Source: CAD feature listing. Evaluate the final solid. Frame: model axes, mm. A direction names the side the tool comes from. Round coordinates to 2 decimals unless told otherwise and drop trailing zeros. Loops run counter-clockwise (first coordinate to the right, second up) from the corner with the lowest first, then second, coordinate; pieces in that order, holes last.
Item 1: Section query B-B on y = 0. Return loops of the section in (x, z), then the cut area to 3 significant figures.
Item 2: Section query C-C on z = -16. Give the number of separate pieces and of enclosed holes in the cut face, then the cut area to 3 significant figures.
Item 3: Access query for faces 4 (the flat face through (10, 71, -21)), 5 (the flat face through (-3.965, 62.6, -27.4)), 6 (the flat face through (0, 3.965, -13)), 7 (the cylindrical face through (14.856, 165.986, -46.208)), 8 (the flat face through (-3.1, 70, -38)). Directions: +Z, -Z, +X, -X, +Y, -Y. A direction counts if a zero-diameter tool reaches every point of the face in a straight line with its end or side. Return the directions, or none.
Item 4: Pull-direction query (Z, two-part tool) for faces 1 (the flat face through (0, 164, -30)), 2 (the flat face through (7, 81, -20)), 3 (the flat face through (7, 10, -10)); classes: released by +Z, released by -Z, zero draft, split by the parting line, or undercut.
Item 5: Ray query, L1, parallel to Y at x = 0, z = -9.5; L2, parallel to Z at x = 9.5, y = 94; L3, parallel to Z at x = 0, y = 91. Return the intervals inside material, ascending.
Item 6: First-contact query: P1, Ø4.5, axis at x = -1, z = -19.5, coming from the +Y side; P2, Ø12, axis at y = 67.5, z = -28.5, coming from the +X side; P3, Ø2, axis at x = -1.5, z = -29.5, coming from the +Y side; P4, Ø21.5, axis at y = 58.5, z = -7, coming from the +X side. Flat tips, straight axial feed; report the tip coordinate or a pass-through.
Item 7: Section query A-A on x = 0. Return loops of the section in (y, z).
```python
from build123d import *

# Parameters (mm, degrees)
SKETCH2_R           = 2.5
SKETCH4_W           = 40
SKETCH4_H           = 40
BOSS_EXTRUDE1_DEPTH = 15
SKETCH5_R           = 10
CUT_EXTRUDE1_DEPTH  = 1
SKETCH6_R           = 2.5
BOSS_EXTRUDE2_DEPTH = 2


with BuildPart() as part:
    # Sweep1: sweep along a path in Sketch3
    with BuildLine(Plane(origin=(0, 0, 0), x_dir=(0, 0, -1), z_dir=(1, 0, 0))) as sweep1_path:
        Line((0, 0), (30, 0))
        Line((30, 0), (30, 150))
    # Sketch2 → Sweep1 (sweep)
    with BuildSketch(Plane.XY):
        with BuildLine():
            Line((-10, -10), (-3.1, -10))
            Line((-3.1, -10), (-3.1, -7.81857447))
            Line((-3.1, -7.81857447), (-4.285374034, -7.81857447))
            ThreePointArc((-4.285374034, -7.81857447), (-5.210402021, -7.198473435), (-4.988208383, -6.107220917))
            Line((-4.988208383, -6.107220917), (-2.819718275, -3.96470075))
            Line((-2.819718275, -3.96470075), (0, -3.96470075))
            Line((0, -3.96470075), (2.782738033, -3.96470075))
            Line((2.782738033, -3.96470075), (5.105242131, -6.103332486))
            ThreePointArc((5.105242131, -6.103332486), (5.359419929, -7.202533996), (4.427854938, -7.838959152))
            Line((4.427854938, -7.838959152), (3.1, -7.838959152))
            Line((3.1, -7.838959152), (3.1, -10))
            Line((3.1, -10), (10, -10))
            Line((10, -10), (10, -3.1))
            Line((10, -3.1), (7.81857447, -3.1))
            Line((7.81857447, -3.1), (7.81857447, -4.285374034))
            ThreePointArc((7.81857447, -4.285374034), (7.198473435, -5.210402021), (6.107220917, -4.988208383))
            Line((6.107220917, -4.988208383), (3.96470075, -2.819718275))
            Line((3.96470075, -2.819718275), (3.96470075, 0))
            Line((3.96470075, 0), (3.96470075, 2.782738033))
            Line((3.96470075, 2.782738033), (6.103332486, 5.105242131))
            ThreePointArc((6.103332486, 5.105242131), (7.202533996, 5.359419929), (7.838959152, 4.427854938))
            Line((7.838959152, 4.427854938), (7.838959152, 3.1))
            Line((7.838959152, 3.1), (10, 3.1))
            Line((10, 3.1), (10, 10))
            Line((10, 10), (3.1, 10))
            Line((3.1, 10), (3.1, 7.81857447))
            Line((3.1, 7.81857447), (4.285374034, 7.81857447))
            ThreePointArc((4.285374034, 7.81857447), (5.210402021, 7.198473435), (4.988208383, 6.107220917))
            Line((4.988208383, 6.107220917), (2.819718275, 3.96470075))
            Line((2.819718275, 3.96470075), (0, 3.96470075))
            Line((0, 3.96470075), (-2.782738033, 3.96470075))
            Line((-2.782738033, 3.96470075), (-5.105242131, 6.103332486))
            ThreePointArc((-5.105242131, 6.103332486), (-5.359419929, 7.202533996), (-4.427854938, 7.838959152))
            Line((-4.427854938, 7.838959152), (-3.1, 7.838959152))
            Line((-3.1, 7.838959152), (-3.1, 10))
            Line((-3.1, 10), (-10, 10))
            Line((-10, 10), (-10, 3.1))
            Line((-10, 3.1), (-7.81857447, 3.1))
            Line((-7.81857447, 3.1), (-7.81857447, 4.285374034))
            ThreePointArc((-7.81857447, 4.285374034), (-7.198473435, 5.210402021), (-6.107220917, 4.988208383))
            Line((-6.107220917, 4.988208383), (-3.96470075, 2.819718275))
            Line((-3.96470075, 2.819718275), (-3.96470075, 0))
            Line((-3.96470075, 0), (-3.96470075, -2.782738033))
            Line((-3.96470075, -2.782738033), (-6.103332486, -5.105242131))
            ThreePointArc((-6.103332486, -5.105242131), (-7.202533996, -5.359419929), (-7.838959152, -4.427854938))
            Line((-7.838959152, -4.427854938), (-7.838959152, -3.1))
            Line((-7.838959152, -3.1), (-10, -3.1))
            Line((-10, -3.1), (-10, -10))
        make_face()
        Circle(SKETCH2_R, mode=Mode.SUBTRACT)
    sweep(path=sweep1_path.line, transition=Transition.RIGHT)

    # Sketch4 → Boss-Extrude1 (add)
    with BuildSketch(Plane(origin=(0, 150, 0), x_dir=(1, 0, 0), z_dir=(0, 1, 0))):
        with Locations((0, 30)):
            Rectangle(SKETCH4_W, SKETCH4_H)
    extrude(amount=BOSS_EXTRUDE1_DEPTH)

    # Sketch5 → Cut-Extrude1 (cut)
    with BuildSketch(Plane(origin=(0, 165, 0), x_dir=(1, 0, 0), z_dir=(0, 1, 0))):
        with Locations(Location((0, 30, 0), (0, 0, 270))):
            Circle(SKETCH5_R)
    extrude(amount=-CUT_EXTRUDE1_DEPTH, mode=Mode.SUBTRACT)

    # Sketch6 → Boss-Extrude2 (add)
    with BuildSketch(Plane(origin=(0, 165, 0), x_dir=(1, 0, 0), z_dir=(0, 1, 0))):
        with Locations(Location((-13.898862729, 43.898862729, 0), (0, 0, 90))):
            Circle(SKETCH6_R)
        with Locations(Location((13.898862729, 43.898862729, 0), (0, 0, 90))):
            Circle(SKETCH6_R)
        with Locations(Location((13.898862729, 16.101137271, 0), (0, 0, 90))):
            Circle(SKETCH6_R)
        with Locations(Location((-13.898862729, 16.101137271, 0), (0, 0, 90))):
            Circle(SKETCH6_R)
    extrude(amount=BOSS_EXTRUDE2_DEPTH)


solid = part.part
```
Data:
1. outline: (-10, -40) - (-3.1, -40) - (-3.1, -37.82) - (-4.29, -37.82) arc R1 cw to (-4.99, -36.11) - (-2.82, -33.96) - (2.78, -33.96) - (5.11, -36.1) arc R1 cw to (4.43, -37.84) - (3.1, -37.84) - (3.1, -40) - (10, -40) - (10, -33.1) - (7.82, -33.1) - (7.82, -34.29) arc R1 cw to (6.11, -34.99) - (3.96, -32.82) - (3.96, 0) - (2.5, 0) - (2.5, -30) arc R2.5 cw to (-2.5, -30) - (-2.5, 0) - (-3.96, 0) - (-3.96, -32.78) - (-6.1, -35.11) arc R1 cw to (-7.84, -34.43) - (-7.84, -33.1) - (-10, -33.1) - close
1. area: 182 mm2
2. separate pieces: 2
2. enclosed holes: 1
2. area: 808 mm2
3. face 4: +Z, -Z, +X, -Y
3. face 5: -X
3. face 6: +Z
3. face 7: +Y
3. face 8: -Z, -Y
4. face 1: undercut
4. face 2: released by +Z
4. face 3: zero draft
5. L1: y = -3.96 to -2.5, 2.5 to 3.96
5. L2: z = -40 to -33.1, -26.9 to -20
5. L3: z = -33.96 to -32.5, -27.5 to -26.04
6. P1: stops at y = 165
6. P2: stops at x = 10
6. P3: stops at y = 164
6. P4: passes through
7. outline: (-3.96, -33.96) - (150, -33.96) - (150, -50) - (165, -50) - (165, -40) - (164, -40) - (164, -20) - (165, -20) - (165, -10) - (150, -10) - (150, -26.04) - (3.96, -26.04) - (3.96, 0) - (2.5, 0) - (2.5, -27.5) - (150, -27.5) - (150, -32.5) - (-2.5, -32.5) - (-2.5, 0) - (-3.96, 0) - close
